```python
from build123d import *

# Parameters (mm, degrees)
SKETCH1_W             = 240
SKETCH1_H             = 50
BOSS_EXTRUDE1_DEPTH   = 25
SKETCH6_OUTSIDE_W     = 291.284
SKETCH6_OUTSIDE_H     = 101.284
SKETCH6_OUTSIDE_W_2   = 236
SKETCH6_OUTSIDE_H_2   = 46
CUT_EXTRUDE3_DEPTH    = 7
CHAMFER6_SIZE         = 3
CHAMFER5_SIZE         = 4
SKETCH6_9_OUTSIDE_W   = 291.284
SKETCH6_9_OUTSIDE_H   = 101.284
SKETCH6_9_OUTSIDE_W_2 = 236
SKETCH6_9_OUTSIDE_H_2 = 46
SKETCH6_9_OUTSIDE_R   = 4.3
CUT_EXTRUDE5_DEPTH    = 3.6
SKETCH16_R            = 2.45
CUT_EXTRUDE10_DEPTH   = 16
CHAMFER8_SIZE         = 0.5
CHAMFER9_SIZE         = 3
CHAMFER9_SIZE2        = 5.196152423
CHAMFER11_SIZE        = 0.5
CHAMFER12_SIZE        = 0.5
CUT_EXTRUDE11_DEPTH   = 20
CHAMFER13_SIZE        = 0.5
CHAMFER14_SIZE        = 3


with BuildPart() as part:
    # Sketch1 → Boss-Extrude1 (new body)
    with BuildSketch(Plane(origin=(0, 0, 0), x_dir=(1, 0, 0), z_dir=(0, 1, 0))):
        with Locations((115, 20)):
            Rectangle(SKETCH1_W, SKETCH1_H)
    extrude(amount=-BOSS_EXTRUDE1_DEPTH)

    # Sketch6 outside → Cut-Extrude3 (cut)
    with BuildSketch(Plane(origin=(0, 0, 0), x_dir=(1, 0, 0), z_dir=(0, 1, 0))):
        with Locations((115, 20)):
            Rectangle(SKETCH6_OUTSIDE_W, SKETCH6_OUTSIDE_H)
        with Locations((115, 20)):
            Rectangle(SKETCH6_OUTSIDE_W_2, SKETCH6_OUTSIDE_H_2, mode=Mode.SUBTRACT)
    extrude(amount=-CUT_EXTRUDE3_DEPTH, mode=Mode.SUBTRACT)

    # Chamfer6
    chamfer6_edges = [part.edges().sort_by_distance(p)[0] for p in [
        (-3, -3.5, -43),
        (233, -3.5, -43),
        (233, -3.5, 3),
        (-3, -3.5, 3),
    ]]
    chamfer(chamfer6_edges, length=CHAMFER6_SIZE)

    # Chamfer5
    chamfer5_edges = [part.edges().sort_by_distance(p)[0] for p in [
        (-5, -16, 5),
        (-5, -16, -45),
        (235, -16, -45),
        (235, -16, 5),
    ]]
    chamfer(chamfer5_edges, length=CHAMFER5_SIZE)

    # Sketch6<9> outside → Cut-Extrude5 (cut)
    # profile 1 of 5: a face of its own
    with BuildSketch(Plane(origin=(0, 0, 0), x_dir=(1, 0, 0), z_dir=(0, 1, 0))):
        with Locations((115, 20)):
            Rectangle(SKETCH6_9_OUTSIDE_W, SKETCH6_9_OUTSIDE_H)
        with Locations((115, 20)):
            Rectangle(SKETCH6_9_OUTSIDE_W_2, SKETCH6_9_OUTSIDE_H_2, mode=Mode.SUBTRACT)
    # profile 2 of 5: a face of its own
    with BuildSketch(Plane(origin=(0, 0, 0), x_dir=(1, 0, 0), z_dir=(0, 1, 0))):
        with Locations(Location((2.7, 37.3, 0), (0, 0, 270))):
            Circle(SKETCH6_9_OUTSIDE_R)
    # profile 3 of 5: a face of its own
    with BuildSketch(Plane(origin=(0, 0, 0), x_dir=(1, 0, 0), z_dir=(0, 1, 0))):
        with Locations(Location((227.3, 37.3, 0), (0, 0, 270))):
            Circle(SKETCH6_9_OUTSIDE_R)
    # profile 4 of 5: a face of its own
    with BuildSketch(Plane(origin=(0, 0, 0), x_dir=(1, 0, 0), z_dir=(0, 1, 0))):
        with Locations(Location((227.3, 2.7, 0), (0, 0, 270))):
            Circle(SKETCH6_9_OUTSIDE_R)
    # profile 5 of 5: a face of its own
    with BuildSketch(Plane(origin=(0, 0, 0), x_dir=(1, 0, 0), z_dir=(0, 1, 0))):
        with Locations(Location((2.7, 2.7, 0), (0, 0, 270))):
            Circle(SKETCH6_9_OUTSIDE_R)
    extrude(amount=-CUT_EXTRUDE5_DEPTH, mode=Mode.SUBTRACT)

    # Sketch16 → Cut-Extrude10 (cut)
    with BuildSketch(Plane(origin=(0, -3.6, 0), x_dir=(1, 0, 0), z_dir=(0, 1, 0))):
        with Locations(Location((2.7, 2.7, 0), (0, 0, 270))):
            Circle(SKETCH16_R)
        with Locations(Location((2.7, 37.3, 0), (0, 0, 270))):
            Circle(SKETCH16_R)
        with Locations(Location((227.3, 37.3, 0), (0, 0, 270))):
            Circle(SKETCH16_R)
        with Locations(Location((227.3, 2.7, 0), (0, 0, 270))):
            Circle(SKETCH16_R)
    extrude(amount=-CUT_EXTRUDE10_DEPTH, mode=Mode.SUBTRACT)

    # Chamfer8
    chamfer8_edges = [part.edges().sort_by_distance(p)[0] for p in [
        (227.3, -3.6, -5.15),
        (227.3, -3.6, -39.75),
        (2.7, -3.6, -39.75),
        (2.7, -3.6, -5.15),
    ]]
    chamfer(chamfer8_edges, length=CHAMFER8_SIZE)

    # Chamfer9
    chamfer9_edges = [part.edges().sort_by_distance(p)[0] for p in [
        (115, -25, -45),
        (-5, -25, -20),
        (115, -25, 5),
        (235, -25, -20),
        (233, -25, -43),
        (233, -25, 3),
        (-3, -25, 3),
        (-3, -25, -43),
    ]]
    chamfer9_side = [part.faces().sort_by_distance(p)[0] for p in [
        (115, -25, -20),
    ]]
    chamfer(chamfer9_edges, length=CHAMFER9_SIZE, length2=CHAMFER9_SIZE2, reference=chamfer9_side[0])

    # Chamfer11
    chamfer11_edges = [part.edges().sort_by_distance(p)[0] for p in [
        (115, 0, 3),
        (-3, 0, -20),
        (233, 0, -20),
        (115, 0, -43),
        (-1.5, 0, 1.5),
        (-1.5, 0, -41.5),
        (231.5, 0, -41.5),
        (231.5, 0, 1.5),
    ]]
    chamfer(chamfer11_edges, length=CHAMFER11_SIZE)

    # Chamfer12
    chamfer12_edges = [part.edges().sort_by_distance(p)[0] for p in [
        (115, -7, -45),
        (115, -7, 5),
        (235, -7, -20),
        (-5, -7, -20),
        (233, -7, -43),
        (233, -7, 3),
        (-3, -7, 3),
        (-3, -7, -43),
    ]]
    chamfer(chamfer12_edges, length=CHAMFER12_SIZE)

    # Sketch18 → Cut-Extrude11 (cut)
    with BuildSketch(Plane(origin=(0, 0, 0), x_dir=(1, 0, 0), z_dir=(0, 1, 0))):
        with BuildLine():
            Line((230, 12.092866172), (230, 27.907133828))
            ThreePointArc((230, 27.907133828), (229.154913652, 29.994320249), (227.095768564, 30.905604835))
            ThreePointArc((227.095768564, 30.905604835), (222.776174185, 32.776174185), (220.905604835, 37.095768564))
            ThreePointArc((220.905604835, 37.095768564), (219.994320249, 39.154913652), (217.907133828, 40))
            Line((217.907133828, 40), (12.092866172, 40))
            ThreePointArc((12.092866172, 40), (10.005679751, 39.154913652), (9.094395165, 37.095768564))
            ThreePointArc((9.094395165, 37.095768564), (7.223825815, 32.776174185), (2.904231436, 30.905604835))
            ThreePointArc((2.904231436, 30.905604835), (0.845086348, 29.994320249), (0, 27.907133828))
            Line((0, 27.907133828), (0, 12.092866172))
            ThreePointArc((0, 12.092866172), (0.845086348, 10.005679751), (2.904231436, 9.094395165))
            ThreePointArc((2.904231436, 9.094395165), (7.223825815, 7.223825815), (9.094395165, 2.904231436))
            ThreePointArc((9.094395165, 2.904231436), (10.005679751, 0.845086348), (12.092866172, 0))
            Line((12.092866172, 0), (217.907133828, 0))
            ThreePointArc((217.907133828, 0), (219.994320249, 0.845086348), (220.905604835, 2.904231436))
            ThreePointArc((220.905604835, 2.904231436), (222.776174185, 7.223825815), (227.095768564, 9.094395165))
            ThreePointArc((227.095768564, 9.094395165), (229.154913652, 10.005679751), (230, 12.092866172))
        make_face()
    extrude(amount=-CUT_EXTRUDE11_DEPTH, mode=Mode.SUBTRACT)

    # Chamfer13
    chamfer13_edges = [part.edges().sort_by_distance(p)[0] for p in [
        (229.154913652, 0, -29.994320249),
        (222.776174185, 0, -32.776174185),
        (219.994320249, 0, -39.154913652),
        (115, 0, -40),
        (10.005679751, 0, -39.154913652),
        (7.223825815, 0, -32.776174185),
        (0.845086348, 0, -29.994320249),
        (0, 0, -20),
        (0.845086348, 0, -10.005679751),
        (7.223825815, 0, -7.223825815),
        (10.005679751, 0, -0.845086348),
        (115, 0, 0),
        (219.994320249, 0, -0.845086348),
        (222.776174185, 0, -7.223825815),
        (229.154913652, 0, -10.005679751),
        (230, 0, -20),
    ]]
    chamfer(chamfer13_edges, length=CHAMFER13_SIZE)

    # Chamfer14
    chamfer14_edges = [part.edges().sort_by_distance(p)[0] for p in [
        (222.776174185, -20, -32.776174185),
        (219.994320249, -20, -39.154913652),
        (115, -20, -40),
        (10.005679751, -20, -39.154913652),
        (7.223825815, -20, -32.776174185),
        (0.845086348, -20, -29.994320249),
        (0, -20, -20),
        (0.845086348, -20, -10.005679751),
        (7.223825815, -20, -7.223825815),
        (10.005679751, -20, -0.845086348),
        (115, -20, 0),
        (219.994320249, -20, -0.845086348),
        (222.776174185, -20, -7.223825815),
        (229.154913652, -20, -10.005679751),
        (230, -20, -20),
        (229.154913652, -20, -29.994320249),
    ]]
    chamfer(chamfer14_edges, length=CHAMFER14_SIZE - 0.0001)  # a hair under: the kernel refuses the full size


solid = part.part
```
Could you check a few things on this model? Use its own coordinates, in mm. A direction names the side the tool comes from. Coordinates: 2 decimals unless noted, no trailing zeros. Loops run counter-clockwise (first coordinate to the right, second up) from the corner with the lowest first, then second, coordinate; pieces in that order, holes last.
1) Thinking about a two-plate mould opening in X: for faces 4 (the face through (232.85, -7.25, 2.8)), 5 (the face through (4, -1.8, -33.2)), 6 (the face through (227, -19.6, -3)), 7 (the face through (-1.926, -22.366, 1.982)), which applies, released by +X, released by -X, zero draft, split by the parting line, or undercut?
Reported:
face 4: released by +X
face 5: undercut
face 6: undercut
face 7: released by -X
2) Please list where these lines run through material, in increasing order: line 1 along X through (y, z) = (-11.75, -2.7); line 2 along X through (y, z) = (-0.8, -2.7); line 3 along Z through (x, y) = (227.3, -11.75).
Reported:
line 1: x = -5 to 0.25, 5.15 to 9.11, 220.89 to 224.85, 229.75 to 235
line 2: x = -3 to -1.6, 7 to 9.11, 220.89 to 223, 231.6 to 233
line 3: z = -45 to -39.75, -34.85 to -30.89, -9.11 to -5.15, -0.25 to 5
3) Will these pins go through, and if not, where does the flat tip stop? pin 1 Ø12 at (x, z) = (71, -12.5) entering from +Y; pin 2 Ø2 at (y, z) = (-4.5, -25) entering from -X; pin 3 Ø8 at (x, z) = (2.7, -37.3) entering from +Y; pin 4 Ø12 at (x, y) = (104.5, -22) entering from +Z.
Reported:
pin 1: stops at y = -20
pin 2: stops at x = -3
pin 3: stops at y = -3.6
pin 4: stops at z = 5
4) Imagine slicing it at B-B (x = 181). List the corners of the cut face in (y, z) for me, and give its area (3 significant figures).
Reported:
outline: (-25, -42) - (-19.8, -45) - (-7.5, -45) - (-7, -44.5) - (-7, -43) - (-0.5, -43) - (0, -42.5) - (0, -40.5) - (-0.5, -40) - (-17, -40) - (-20, -37) - (-20, -3) - (-17, 0) - (-0.5, 0) - (0, 0.5) - (0, 2.5) - (-0.5, 3) - (-7, 3) - (-7, 4.5) - (-7.5, 5) - (-19.8, 5) - (-25, 2) - close
area: 415 mm2
5) Imagine slicing it at A-A (z = -22). List the corners of the cut face in (x, y) for me, and give its area (3 significant figures).
Reported:
outline: (-5, -19.8) - (-2, -25) - (232, -25) - (235, -19.8) - (235, -7.5) - (234.5, -7) - (233, -7) - (233, -0.5) - (232.5, 0) - (230.5, 0) - (230, -0.5) - (230, -17) - (227, -20) - (3, -20) - (0, -17) - (0, -0.5) - (-0.5, 0) - (-2.5, 0) - (-3, -0.5) - (-3, -7) - (-4.5, -7) - (-5, -7.5) - close
area: 1,360 mm2
6) Which directions (+Z, -Z, +X, -X, +Y, -Y) give clear straight access to the entire face, cutting with the end or side of a thin tool? Please do faces 1 (the face through (113, -4, 3)), 2 (the face through (113, -20, -20)), 3 (the face through (113, -4, -43)).
Reported:
face 1: +Z, +X, -X, +Y
face 2: +Y
face 3: -Z, +X, -X, +Y
